For this review, take the finished solid that the model builds, in its own axes (mm). Round coordinates to 2 decimals unless told otherwise and drop trailing zeros. Loops run counter-clockwise (first coordinate to the right, second up) from the corner with the lowest first, then second, coordinate; pieces in that order, holes last. Notation, with made-up numbers: (62.5, -8.5) -> (81.5, -8.5) arc R11 cw to (81.5, 5.5) -> close; hole circle Ø11 at (58, 75). An arc over 180 degrees is marked (long way). Use one line per item in the form item = value. Start each with the question number.
from build123d import *

# Parameters (mm, degrees)
SKETCH1_W               = 14
SKETCH1_H               = 6
BOSS_EXTRUDE1_DEPTH     = 4
CUT_EXTRUDE1_DEPTH      = 16.748015748
CUT_EXTRUDE1_DEPTH_BACK = 16.748015748
SKETCH2_R               = 1.15
SKETCH2_R_2             = 1.45
FILLET1_R               = 3


with BuildPart() as part:
    # Sketch1 → Boss-Extrude1 (new body)
    with BuildSketch(Plane.XY):
        with Locations((7, -3)):
            Rectangle(SKETCH1_W, SKETCH1_H)
    extrude(amount=BOSS_EXTRUDE1_DEPTH)

    # Sketch2 → Cut-Extrude1 (cut, two sides: drawn at the far end of the back side and taken through both)
    with BuildSketch(Plane.XY.offset(4).offset(-CUT_EXTRUDE1_DEPTH_BACK)):
        with Locations((3, -3)):
            Circle(SKETCH2_R)
        with Locations((11, -3)):
            Circle(SKETCH2_R_2)
    extrude(amount=CUT_EXTRUDE1_DEPTH + CUT_EXTRUDE1_DEPTH_BACK, mode=Mode.SUBTRACT)

    # Fillet1
    fillet1_edges = [part.edges().sort_by_distance(p)[0] for p in [
        (14, -6, 2),
        (14, 0, 2),
        (0, -6, 2),
        (0, 0, 2),
    ]]
    fillet(fillet1_edges, radius=FILLET1_R - 0.0001)  # a hair under: the kernel refuses the full size


solid = part.part
Item 1: Take a section at B-B on y = -2.15. Give the boundary of the cut face in (x, z).
Item 2: For P1, Ø1.8, axis at x = 3, y = -3, coming from the -Z side, flat-tipped, find the tip position at first contact; note if it passes through.
Item 3: Wall thickness on line 1 (X direction, y = -3, z = 2); line 2 (Y direction, x = 11, z = 3.25); line 3 (Y direction, x = 3, z = 2.3): over which ranges is each line inside the solid? List them lowest first.
Item 4: Take a section at C-C on x = 11.5. Give the boundary of the cut face in (y, z), plus the area to 3 significant figures.
Item 5: Take a section at A-A on z = 3.35. Give the number of separate pieces and of enclosed holes in the cut face, plus the area to 3 significant figures.
Item 6: Take a section at D-D on x = 2. Give the boundary of the cut face in (y, z).
Item 7: Draft analysis for pull direction X (two halves, no side actions). For faces 1 (the cylindrical face through (2.751, -4.123, 1.972)), 2 (the flat face through (7, 0, 2)), 3 (the cylindrical face through (0.86, -0.9, 2.03)), 4 (the cylindrical face through (9.55, -2.94, 1.97)), state which applies: +X half, -X half, draft (parallel to the pull), parting line (faces both ways), or undercut.
Results:
q1.outline = (0.12, 0) -> (2.23, 0) -> (2.23, 4) -> (0.12, 4) -> close; (3.77, 0) -> (9.83, 0) -> (9.83, 4) -> (3.77, 4) -> close; (12.17, 0) -> (13.88, 0) -> (13.88, 4) -> (12.17, 4) -> close
q2.P1 = through
q3.line_1 = 0 to 1.85, 4.15 to 9.55, 12.45 to 14
q3.line_2 = -6 to -4.45, -1.55 to 0
q3.line_3 = -6 to -4.15, -1.85 to 0
q4.outline = (-5.96, 0) -> (-4.36, 0) -> (-4.36, 4) -> (-5.96, 4) -> close; (-1.64, 0) -> (-0.04, 0) -> (-0.04, 4) -> (-1.64, 4) -> close
q4.area = 12.8 mm2
q5.separate_pieces = 1
q5.enclosed_holes = 2
q5.area = 65.5 mm2
q6.outline = (-5.83, 0) -> (-3.57, 0) -> (-3.57, 4) -> (-5.83, 4) -> close; (-2.43, 0) -> (-0.17, 0) -> (-0.17, 4) -> (-2.43, 4) -> close
q7.face_1 = undercut
q7.face_2 = draft
q7.face_3 = -X half
q7.face_4 = undercut
